```python
from build123d import *


with BuildPart() as part:
    # Sketch2 → Revolve2 (revolve)
    with BuildSketch(Plane.XY, mode=Mode.PRIVATE) as revolve2_sk:
        with BuildLine():
            Line((0, 168.903192951), (15, 168.903192951))
            Line((15, 168.903192951), (15, 150.903192951))
            Line((15, 150.903192951), (16.6, 150.903192951))
            Line((16.6, 150.903192951), (16.6, 148.903192951))
            Line((16.6, 148.903192951), (13.5, 148.903192951))
            add(Edge.make_bspline(
                [(13.5, 148.903192951), (13.434542306, 147.062564488), (13.708566417, 145.26063883), (14.322072332, 143.497415977)],
                knots=[0, 0, 0, 0, 1, 1, 1, 1], degree=3))
            Line((14.322072332, 143.497415977), (31.45, 94.271560556))
            add(Edge.make_bspline(
                [(31.45, 94.271560556), (33.229126476, 90.845001817), (26.551628462, 62.433806412), (26.823939199, 27.642446291), (26.534878828, -7.980277801), (29.779872762, -21.167076085), (32.957402386, -29.251025192), (32.695362988, -40.354526378), (31.042317735, -50.939796111), (22.16798563, -63.145599506), (13.030739968, -58.723683942), (6.82762256, -55.368152541), (1.956337431, -55.2690346), (0, -55.33481547)],
                knots=[0, 0, 0, 0, 0.05780284, 0.472965333, 0.582837644, 0.639270184, 0.696109455, 0.72354797, 0.819702818, 0.882564852, 0.920543744, 0.968756394, 1, 1, 1, 1], degree=3))
            Line((0, -55.33481547), (0, 168.903192951))
        make_face()
    revolve(revolve2_sk.sketch.rotate(Axis((0, 168.903192951, 0), (0, -1, 0)), 180), axis=Axis((0, 168.903192951, 0), (0, -1, 0)))


solid = part.part
```
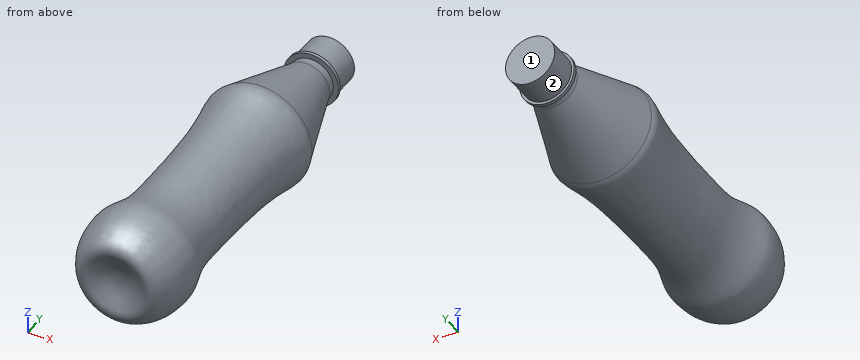
For this review, take the finished solid that the model builds, in its own axes (mm). Face numbers are marked on the shaded views. A direction names the side the tool comes from. Coordinates: 2 decimals unless noted, no trailing zeros.
(1) Tool access review of the marked faces 1 and 2: name each direction out of +Z, -Z, +X, -X, +Y, -Y from which nothing blocks a thin tool from reaching the whole face with its end or side.
(2) Wall thickness on probe 1 along X at (y, z) = (84.5, -28.5); probe 2 along X at (y, z) = (-26, 29); probe 3 along Z at (x, y) = (-18.5, 61.5): over which ranges is each line inside the solid? List them lowest first.
(3) For pin 1 Ø8 at (x, z) = (3.5, 9) entering from -Y; pin 2 Ø2 at (y, z) = (-3, -22) entering from +X; pin 3 Ø10 at (y, z) = (-20, 5.5) entering from -X; pin 4 Ø12 at (x, z) = (19, -1) entering from -Y, all flat-tipped, find the tip position at first contact; note any pin that passes through.
Answer sheet:
1. face 1: +Z, -Z, +X, -X, +Y
1. face 2: +Y
2. probe 1: x = -14.16 to 14.16
2. probe 2: x = -12.53 to 12.53
2. probe 3: z = -21.51 to 21.51
3. pin 1: stops at y = -58.97
3. pin 2: stops at x = 16.65
3. pin 3: stops at x = -30.95
3. pin 4: stops at y = -61.12
